For this review, take the finished solid that the model builds, in its own axes (mm). Give positions to 0.01 mm unless a question says otherwise; leave off trailing zeros. Order: outer loops, then holes, each group sorted by start corner. A loop starts at its lowest first (then second) coordinate and runs counter-clockwise, first axis right, second up.
Item 1: For P1, Ø4, axis at x = 5, z = -9, coming from the -Y side; P2, Ø4, axis at x = 2.5, z = -12, coming from the -Y side; P3, Ø2, axis at x = 4, z = -5.5, coming from the -Y side, all flat-tipped, find the tip position at first contact; note any pin that passes through.
Item 2: Consider section B-B (y = -49.11). Give the boundary of the cut face in (x, z).
Item 3: For probe 1 along Y at (x, z) = (1.5, -8); probe 2 along Z at (x, y) = (4.5, -60); probe 3 along Z at (x, y) = (3.5, -54.5), list the stretches that pass through material, from the lowest coordinate up.
Item 4: Consider section A-A (z = 0). Give the boundary of the cut face in (x, y), plus the area to 3 significant figures.
```python
from build123d import *

# Parameters (mm, degrees)
CHAMFER1_SIZE  = 0.3
CHAMFER2_SIZE  = 0.3
CHAMFER2_SIZE2 = 0.234981042


with BuildPart() as part:
    # Sketch1 → Revolve2 (revolve)
    with BuildSketch(Plane.XY, mode=Mode.PRIVATE) as revolve2_sk:
        with BuildLine():
            Line((0, 0), (7, 0))
            Line((7, 0), (7, 4))
            Line((7, 4), (3.51, 4))
            Line((3.51, 4), (1, 4.89))
            Line((1, 4.89), (1, 4.3766025))
            ThreePointArc((1, 4.3766025), (1.086926266, 4.094875522), (1.317480361, 3.911106441))
            Line((1.317480361, 3.911106441), (4.292031423, 2.744793695))
            ThreePointArc((4.292031423, 2.744793695), (4.786077272, 1.851398109), (4, 1.2))
            Line((4, 1.2), (0, 1))
            Line((0, 1), (0, 0))
        make_face()
    revolve(revolve2_sk.sketch.rotate(Axis((7, -49.11, 0), (-1, 0, 0)), 90), axis=Axis((7, -49.11, 0), (-1, 0, 0)))

    # Chamfer1
    chamfer1_edges = [part.edges().sort_by_distance(p)[0] for p in [
        (7, -49.11, 53.11),
    ]]
    chamfer(chamfer1_edges, length=CHAMFER1_SIZE)

    # Chamfer2
    chamfer2_edges = [part.edges().sort_by_distance(p)[0] for p in [
        (1, -49.11, 54),
    ]]
    chamfer2_side = [part.faces().sort_by_distance(p)[0] for p in [
        (1, -49.11, 53.847264935),
    ]]
    chamfer(chamfer2_edges, length=CHAMFER2_SIZE, length2=CHAMFER2_SIZE2, reference=chamfer2_side[0])


solid = part.part
```
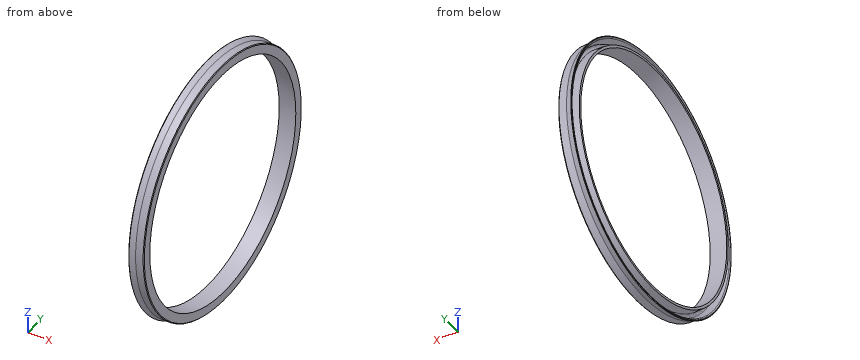
Resolved:
1. P1: stops at y = -101.76
1. P2: stops at y = -102.01
1. P3: stops at y = -102.13
2. outline: (0, -50.11) - (4, -50.31) arc R0.8 cw to (4.29, -51.85) - (1.32, -53.02) arc R0.5 ccw to (1, -53.49) - (1, -53.7) - (1.22, -53.92) - (3.51, -53.11) - (6.7, -53.11) - (7, -52.81) - (7, -49.11) - (0, -49.11) - close; (0, 49.11) - (7, 49.11) - (7, 52.81) - (6.7, 53.11) - (3.51, 53.11) - (1.22, 53.92) - (1, 53.7) - (1, 53.49) arc R0.5 ccw to (1.32, 53.02) - (4.29, 51.85) arc R0.8 cw to (4, 50.31) - (0, 50.11) - close
3. probe 1: y = -102.33 to -101.45, -98.65 to -97.56, -0.66 to 0.43, 3.23 to 4.11
3. probe 2: z = -51.98 to -50.58, -49.3 to -47.89, 47.89 to 49.3, 50.58 to 51.98
3. probe 3: z = -52.84 to -51.89, -50 to -48.81, 48.81 to 50, 51.89 to 52.84
4. outline: (0, -99.22) - (4, -99.42) arc R0.8 cw to (4.29, -100.96) - (1.32, -102.13) arc R0.5 ccw to (1, -102.6) - (1, -102.81) - (1.22, -103.03) - (3.51, -102.22) - (6.7, -102.22) - (7, -101.92) - (7, -98.22) - (0, -98.22) - close; (0, 0) - (7, 0) - (7, 3.7) - (6.7, 4) - (3.51, 4) - (1.22, 4.81) - (1, 4.59) - (1, 4.38) arc R0.5 ccw to (1.32, 3.91) - (4.29, 2.74) arc R0.8 cw to (4, 1.2) - (0, 1) - close
4. area: 36.1 mm2
